```python
from build123d import *

# Parameters (mm, degrees)
SKETCH1_R               = 10
BOSS_EXTRUDE1_DEPTH     = 5
SKETCH2_R               = 5
BOSS_EXTRUDE2_DEPTH     = 4
CUT_EXTRUDE1_DEPTH      = 3
CUT_EXTRUDE_THIN1_DEPTH = 5


with BuildPart() as part:
    # Sketch1 → Boss-Extrude1 (new body)
    with BuildSketch(Plane.XY):
        Circle(SKETCH1_R)
    extrude(amount=BOSS_EXTRUDE1_DEPTH)

    # Sketch2 → Boss-Extrude2 (add)
    with BuildSketch(Plane.XY.offset(5)):
        Circle(SKETCH2_R)
    extrude(amount=BOSS_EXTRUDE2_DEPTH)

    # Sketch3 → Cut-Extrude1 (cut)
    with BuildSketch(Plane.XY.offset(9)):
        Polygon((2.048231561, -3.749410728), (4.27120072, -0.1008848), (2.222969159, 3.648525928), (-2.048231561, 3.749410728), (-4.27120072, 0.1008848), (-2.222969159, -3.648525928), align=None)
    extrude(amount=-CUT_EXTRUDE1_DEPTH, mode=Mode.SUBTRACT)

    # Sketch4 → Cut-Extrude-Thin1 (cut)
    with BuildSketch(Plane.XY.offset(5)):
        with BuildLine():
            ThreePointArc((-6.614378278, 7.5), (0, 6.223611165), (6.614378278, 7.5))
            Line((6.614378278, 7.5), (2.893499791, 16.781975183))
            ThreePointArc((2.893499791, 16.781975183), (0, 16.223611165), (-2.893499791, 16.781975183))
            Line((-2.893499791, 16.781975183), (-6.614378278, 7.5))
        make_face()
        with BuildLine():
            ThreePointArc((9.802379667, 1.978219619), (5.389805372, -3.111805583), (3.18800139, -9.478219619))
            Line((3.18800139, -9.478219619), (13.086866938, -10.896831917))
            ThreePointArc((13.086866938, -10.896831917), (14.05005941, -8.111805583), (15.98036673, -5.885143266))
            Line((15.98036673, -5.885143266), (9.802379667, 1.978219619))
        make_face()
        with BuildLine():
            ThreePointArc((-3.18800139, -9.478219619), (-5.389805372, -3.111805583), (-9.802379667, 1.978219619))
            Line((-9.802379667, 1.978219619), (-15.98036673, -5.885143266))
            ThreePointArc((-15.98036673, -5.885143266), (-14.05005941, -8.111805583), (-13.086866938, -10.896831917))
            Line((-13.086866938, -10.896831917), (-3.18800139, -9.478219619))
        make_face()
    extrude(amount=-CUT_EXTRUDE_THIN1_DEPTH, mode=Mode.SUBTRACT)


solid = part.part
```
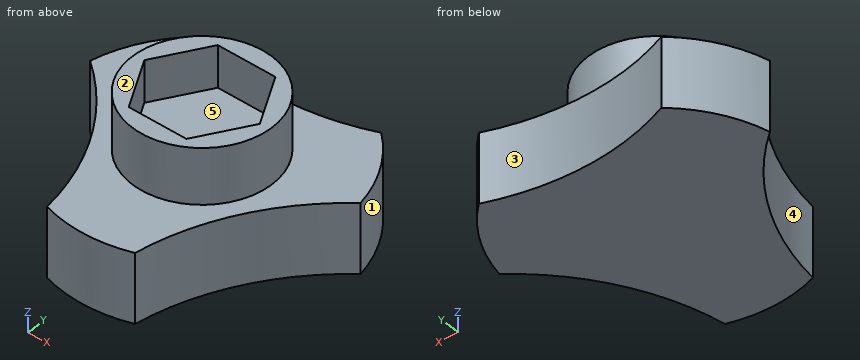
Build history of the part. All positions in model axes, mm. Face numbers are marked on the shaded views. A direction names the side the tool comes from. Round coordinates to 2 decimals unless told otherwise and drop trailing zeros. Loops run counter-clockwise (first coordinate to the right, second up) from the corner with the lowest first, then second, coordinate; pieces in that order, holes last.
Item 1: Saw through at A-A (z = 8.25). List the corners of the cut face in (x, y).
Item 2: Pin check, flat tips, straight feed: P1, Ø1, axis at x = -1, z = 6.5, coming from the -Y side; P2, Ø1.5, axis at y = -2.5, z = 3.5, coming from the -X side. Stop position of each tip, or through.
Item 3: Saw through at B-B (x = 3.75). List the corners of the cut face in (y, z).
Item 4: Saw through at D-D (y = -9). List the corners of the cut face in (x, z), then the cut area to 3 significant figures.
Item 5: Saw through at C-C (z = 3). List the corners of the cut face in (x, y).
Item 6: Two-plate mould, pull along X, no slides. Class the marked faces 1, 2 and 3: released by +X, released by -X, zero draft, split by the parting line, or undercut.
Item 7: Drill centre lines: line 1 along Z through (x, y) = (5.75, 0.5); line 2 along Z through (x, y) = (2, 3.5); line 3 along Y through (x, z) = (-1.5, 6.25). Where is each one in solid material? Low to high.
Item 8: Which spindle directions (+Z, -Z, +X, -X, +Y, -Y) get a long thin tool onto all of the face, cutting with end or side? Do the marked faces 4 and 5. Say none if no direction does.
Worked answers:
1. outline: circle Ø10 at (0, 0); hole (-4.27, 0.1) - (-2.22, -3.65) - (2.05, -3.75) - (4.27, -0.1) - (2.22, 3.65) - (-2.05, 3.75) - close
2. P1: stops at y = -4.97
2. P2: stops at x = -6.26
3. outline: (-6.92, 0) - (6.62, 0) - (6.62, 5) - (3.31, 5) - (3.31, 9) - (0.85, 9) - (0.85, 6) - (-0.96, 6) - (-0.96, 9) - (-3.31, 9) - (-3.31, 5) - (-6.92, 5) - close
4. outline: (-3.26, 0) - (3.26, 0) - (3.26, 5) - (-3.26, 5) - close
4. area: 32.6 mm2
5. outline: (-9.8, 1.98) arc R17.78 cw to (-3.19, -9.48) arc R10 ccw to (3.19, -9.48) arc R17.78 cw to (9.8, 1.98) arc R10 ccw to (6.61, 7.5) arc R17.78 cw to (-6.61, 7.5) arc R10 ccw to start
6. face 1: released by +X
6. face 2: zero draft
6. face 3: undercut
7. line 1: z = 0 to 5
7. line 2: z = 0 to 6
7. line 3: y = -4.77 to -3.67, 3.74 to 4.77
8. face 4: +Z, -Z, -X, -Y
8. face 5: +Z
